```python
from build123d import *

# Parameters (mm, degrees)
SKETCH1_W           = 29
SKETCH1_H           = 29
BOSS_EXTRUDE1_DEPTH = 30
SKETCH2_R           = 14.5
SKETCH2_R_2         = 13
BOSS_EXTRUDE2_DEPTH = 11.76
SKETCH4_W           = 20.6
SKETCH4_H           = 13.6
CUT_EXTRUDE1_DEPTH  = 2
FILLET1_R           = 3
FILLET2_R           = 1
SKETCH5_R           = 3.5
SKETCH5_R_2         = 2.5
BOSS_EXTRUDE3_DEPTH = 8
SKETCH6_R           = 1
CUT_EXTRUDE2_DEPTH  = 3
SKETCH8_R           = 1.5
SKETCH8_R_2         = 1
CUT_EXTRUDE3_DEPTH  = 2
SKETCH9_W           = 22
SKETCH9_H           = 6
BOSS_EXTRUDE4_DEPTH = 1
SKETCH10_R          = 1
CUT_EXTRUDE4_DEPTH  = 2


with BuildPart() as part:
    # Sketch1 → Boss-Extrude1 (new body)
    with BuildSketch(Plane.XY):
        with Locations((-0.780453258, -3.943342776)):
            Rectangle(SKETCH1_W, SKETCH1_H)
    extrude(amount=BOSS_EXTRUDE1_DEPTH)

    # Sketch2 → Boss-Extrude2 (add)
    with BuildSketch(Plane.XY.offset(30)):
        with Locations((-0.780453258, -3.943342776)):
            Circle(SKETCH2_R)
        with Locations((-0.780453258, -3.943342776)):
            Circle(SKETCH2_R_2, mode=Mode.SUBTRACT)
    extrude(amount=BOSS_EXTRUDE2_DEPTH)

    # Sketch4 → Cut-Extrude1 (cut)
    with BuildSketch(Plane.XY.offset(30)):
        with Locations((-0.780453258, -3.943342776)):
            Rectangle(SKETCH4_W, SKETCH4_H)
    extrude(amount=-CUT_EXTRUDE1_DEPTH, mode=Mode.SUBTRACT)

    # Fillet1
    fillet1_edges = [part.edges().sort_by_distance(p)[0] for p in [
        (-11.080453258, -10.743342776, 29),
        (-11.080453258, 2.856657224, 29),
        (9.519546742, 2.856657224, 29),
        (9.519546742, -10.743342776, 29),
    ]]
    fillet(fillet1_edges, radius=FILLET1_R)

    # Fillet2
    fillet2_edges = [part.edges().sort_by_distance(p)[0] for p in [
        (-0.780453258, -10.743342776, 30),
        (-11.080453258, -3.943342776, 30),
        (9.519546742, -3.943342776, 30),
        (-0.780453258, 2.856657224, 30),
        (-10.201773601, -9.86466312, 30),
        (8.640867086, -9.86466312, 30),
        (8.640867086, 1.977977567, 30),
        (-10.201773601, 1.977977567, 30),
    ]]
    fillet(fillet2_edges, radius=FILLET2_R)

    # Sketch5 → Boss-Extrude3 (add)
    with BuildSketch(Plane(origin=(0, 0, 0), x_dir=(-1, 0, 0), z_dir=(0, 0, -1))):
        with Locations((-8.719546742, 5.556657224)):
            Circle(SKETCH5_R)
        with Locations((-8.719546742, 5.556657224)):
            Circle(SKETCH5_R_2, mode=Mode.SUBTRACT)
    extrude(amount=BOSS_EXTRUDE3_DEPTH)

    # Sketch6 → Cut-Extrude2 (cut)
    with BuildSketch(Plane(origin=(0, 10.556657224, 0), x_dir=(1, 0, 0), z_dir=(0, 1, 0))):
        with Locations((-6.780453258, -28)):
            Circle(SKETCH6_R)
        with Locations((5.219546742, -28)):
            Circle(SKETCH6_R)
    extrude(amount=-CUT_EXTRUDE2_DEPTH, mode=Mode.SUBTRACT)

    # Sketch8 → Cut-Extrude3 (cut)
    with BuildSketch(Plane.XZ.offset(18.443342776)):
        with Locations((9.219546742, 27)):
            Circle(SKETCH8_R)
        with Locations((-10.780453258, 27)):
            Circle(SKETCH8_R)
        with Locations((-6.780453258, 25.5)):
            Circle(SKETCH8_R_2)
        with Locations((5.219546742, 25.5)):
            Circle(SKETCH8_R_2)
        with Locations((-6.780453258, 3.5)):
            Circle(SKETCH8_R_2)
        with Locations((5.219546742, 3.5)):
            Circle(SKETCH8_R_2)
        with Locations((-0.780453258, 3.5)):
            Circle(SKETCH8_R)
        with BuildLine():
            Line((-12.280453258, 22.292576019), (10.719546742, 22.292576019))
            ThreePointArc((10.719546742, 22.292576019), (11.426653523, 21.999682801), (11.719546742, 21.292576019))
            Line((11.719546742, 21.292576019), (11.719546742, 7.292576019))
            ThreePointArc((11.719546742, 7.292576019), (11.426653523, 6.585469238), (10.719546742, 6.292576019))
            Line((10.719546742, 6.292576019), (-12.280453258, 6.292576019))
            ThreePointArc((-12.280453258, 6.292576019), (-12.987560039, 6.585469238), (-13.280453258, 7.292576019))
            Line((-13.280453258, 7.292576019), (-13.280453258, 21.292576019))
            ThreePointArc((-13.280453258, 21.292576019), (-12.987560039, 21.999682801), (-12.280453258, 22.292576019))
        make_face()
    extrude(amount=-CUT_EXTRUDE3_DEPTH, mode=Mode.SUBTRACT)

    # Sketch9 → Boss-Extrude4 (add)
    with BuildSketch(Plane(origin=(0, 0, 0), x_dir=(-1, 0, 0), z_dir=(0, 0, -1))):
        with Locations((1.280453258, -13.443342776)):
            Rectangle(SKETCH9_W, SKETCH9_H)
    extrude(amount=BOSS_EXTRUDE4_DEPTH)

    # Sketch10 → Cut-Extrude4 (cut)
    with BuildSketch(Plane(origin=(0, 0, -1), x_dir=(-1, 0, 0), z_dir=(0, 0, -1))):
        with Locations((-7.719546742, -13.443342776)):
            Circle(SKETCH10_R)
        with Locations((10.280453258, -13.443342776)):
            Circle(SKETCH10_R)
    extrude(amount=-CUT_EXTRUDE4_DEPTH, mode=Mode.SUBTRACT)


solid = part.part
```
Here's how the part is built. I have some questions about the finished solid (model axes, mm). A direction names the side the tool comes from. Round coordinates to 2 decimals unless told otherwise and drop trailing zeros. Order: outer loops, then holes, each group sorted by start corner. A loop starts at its lowest first (then second) coordinate and runs counter-clockwise, first axis right, second up. Notation, with made-up numbers: M 29,66.5 L 77,66.5 A35 ccw 77,102.5 Z; hole C 28,-30.5 d5. An arc over 180 degrees is marked long. Use CSV: the item, a comma, the result in double quotes.
1) I want a section at A-A (z = 3.5). List the corners of the cut face in (x, y) for me, then the cut area to 3 significant figures.
Taken from the geometry:
outline,"M -15.28,-18.44 L -7.78,-18.44 L -7.78,-16.44 L -5.78,-16.44 L -5.78,-18.44 L -2.28,-18.44 L -2.28,-16.44 L 0.72,-16.44 L 0.72,-18.44 L 4.22,-18.44 L 4.22,-16.44 L 6.22,-16.44 L 6.22,-18.44 L 13.72,-18.44 L 13.72,10.56 L -15.28,10.56 Z"
area,"827 mm^2"
2) I want a section at D-D (y = 7). List the corners of the cut face in (x, z) for me.
Taken from the geometry:
outline,"M -15.28,0 L 5.53,0 L 5.53,-8 L 6.68,-8 L 6.68,0 L 10.76,0 L 10.76,-8 L 11.91,-8 L 11.91,0 L 13.72,0 L 13.72,30 L 8.73,30 L 8.73,41.76 L 6.24,41.76 L 6.24,30 L -7.8,30 L -7.8,41.76 L -10.29,41.76 L -10.29,30 L -15.28,30 Z"
3) If we mould it in two halves opening along X, with no side actions, what happens to faces 1 (the flat face through (10, 8, 30)), 2 (the flat face through (5, -16.443, 4)), 3 (the flat face through (-13.28, -17, 14))? For each: pulls with the +X half, pulls with the -X half, needs draft (parallel to the pull), parting line crosses it, or undercut.
Taken from the geometry:
face 1,"needs draft"
face 2,"undercut"
face 3,"undercut"
4) I'm going to push flat-ended pins straight in: P1, Ø1, axis at x = 1.5, y = 3, coming from the -Z side; P2, Ø4, axis at x = 2, z = 12, coming from the -Y side; P3, Ø3, axis at y = 7, z = 32, coming from the +X side; P4, Ø3.5, axis at x = -0.78, z = 3.5, coming from the -Y side. Where does each tip first touch, or does it pass through?
Taken from the geometry:
P1,"z = 0"
P2,"y = -16.44"
P3,"x = 10.22"
P4,"y = -18.44"
5) I need wall thicknesses on line 1 along X through (y, z) = (8.7, 28); line 2 along Y through (x, z) = (1.5, 14); line 3 along Z through (x, y) = (-13, 8.5). Which ranges of each line are inside material? Lowest first, please. Write a range as [from, to].
Taken from the geometry:
line 1,"[-15.28, -7.78], [-5.78, 4.22], [6.22, 13.72]"
line 2,"[-16.44, 10.56]"
line 3,"[0, 30]"
6) On a 3-axis mill with a long thin cutter (end or side, diameter ignored), from which of +Z, -Z, +X, -X, +Y, -Y can I reach the whole of each face in a straight line? I mean faces 4 (the cylindrical face through (-5.827, -17.457, 3.8)), 5 (the flat face through (9, 6, 0)), 6 (the flat face through (-1.1, -16.443, -0.5)), 7 (the flat face through (-7, 7.557, 28)), 8 (the cylindrical face through (9.82, -3.89, 29.715)). Say none if no direction works.
Taken from the geometry:
face 4,"-Y"
face 5,"-Z"
face 6,"-Z, +X, -X, -Y"
face 7,"+Y"
face 8,"+Z"
7) I want a section at C-C (z = 16.5). List the corners of the cut face in (x, y) for me, then the cut area to 3 significant figures.
Taken from the geometry:
outline,"M -15.28,-18.44 L -13.28,-18.44 L -13.28,-16.44 L 11.72,-16.44 L 11.72,-18.44 L 13.72,-18.44 L 13.72,10.56 L -15.28,10.56 Z"
area,"791 mm^2"
